```python
from build123d import *

# Parameters (mm, degrees)
CROQUIS1_W              = 167.894
CROQUIS1_H              = 52.07
SALIENTE_EXTRUIR1_DEPTH = 25.4
CROQUIS2_W              = 35
CROQUIS2_H              = 48.57
CORTAR_EXTRUIR1_DEPTH   = 25.4
CORTAR_EXTRUIR2_DEPTH   = 25.4
REDONDEO1_R             = 5
REDONDEO2_R             = 5
REDONDEO6_R             = 5
REDONDEO7_R             = 5
REDONDEO11_R            = 5
REDONDEO12_R            = 5
REDONDEO13_R            = 5
CROQUIS4_R              = 1.5
CORTAR_EXTRUIR3_DEPTH   = 76.2


with BuildPart() as part:
    # Croquis1 → Saliente-Extruir1 (new body)
    with BuildSketch(Plane.XY):
        with Locations((-83.947, 26.035)):
            Rectangle(CROQUIS1_W, CROQUIS1_H)
    extrude(amount=SALIENTE_EXTRUIR1_DEPTH)

    # Croquis2 → Cortar-Extruir1 (cut)
    with BuildSketch(Plane.XY.offset(25.4)):
        Polygon((-119.137953593, 52.07), (-132.894, 52.07), (-132.894, 3.5), (-120.129227268, 48.57), align=None)
        with Locations((-150.394, 27.785)):
            Rectangle(CROQUIS2_W, CROQUIS2_H)
        with Locations((-17.5, 27.785)):
            Rectangle(CROQUIS2_W, CROQUIS2_H)
        Polygon((-35, 52.07), (-48.756046407, 52.07), (-47.764772732, 48.57), (-35, 3.5), align=None)
    extrude(amount=-CORTAR_EXTRUIR1_DEPTH, mode=Mode.SUBTRACT)

    # Croquis3 → Cortar-Extruir2 (cut)
    with BuildSketch(Plane.XY.offset(25.4)):
        Polygon((-117.509109836, 48.57), (-50.384890164, 48.57), (-38.5, 3.5), (-38.5, 0), (-129.394, 0), (-129.394, 3.5), align=None)
    extrude(amount=-CORTAR_EXTRUIR2_DEPTH, mode=Mode.SUBTRACT)

    # Redondeo1
    redondeo1_edges = [part.edges().sort_by_distance(p)[0] for p in [
        (-48.756046407, 52.07, 12.7),
    ]]
    fillet(redondeo1_edges, radius=REDONDEO1_R)

    # Redondeo2
    redondeo2_edges = [part.edges().sort_by_distance(p)[0] for p in [
        (-119.137953593, 52.07, 12.7),
    ]]
    fillet(redondeo2_edges, radius=REDONDEO2_R)

    # Redondeo6
    redondeo6_edges = [part.edges().sort_by_distance(p)[0] for p in [
        (-38.5, 3.5, 12.7),
    ]]
    fillet(redondeo6_edges, radius=REDONDEO6_R)

    # Redondeo7
    redondeo7_edges = [part.edges().sort_by_distance(p)[0] for p in [
        (-129.394, 3.5, 12.7),
    ]]
    fillet(redondeo7_edges, radius=REDONDEO7_R)

    # Redondeo11
    redondeo11_edges = [part.edges().sort_by_distance(p)[0] for p in [
        (-129.394, 0, 12.7),
    ]]
    fillet(redondeo11_edges, radius=REDONDEO11_R)

    # Redondeo12
    redondeo12_edges = [part.edges().sort_by_distance(p)[0] for p in [
        (-38.5, 0, 12.7),
    ]]
    fillet(redondeo12_edges, radius=REDONDEO12_R)

    # Redondeo13
    redondeo13_edges = [part.edges().sort_by_distance(p)[0] for p in [
        (-132.894, 3.5, 12.7),
        (-35, 3.5, 12.7),
    ]]
    fillet(redondeo13_edges, radius=REDONDEO13_R)

    # Croquis4 → Cortar-Extruir3 (cut)
    with BuildSketch(Plane(origin=(0, 52.07, 0), x_dir=(1, 0, 0), z_dir=(0, 1, 0))):
        with Locations((-157.894, -5)):
            Circle(CROQUIS4_R)
        with Locations((-146.674562343, -20.4)):
            Circle(CROQUIS4_R)
        with Locations((-21.219437657, -20.4)):
            Circle(CROQUIS4_R)
        with Locations((-10, -5)):
            Circle(CROQUIS4_R)
    extrude(amount=-CORTAR_EXTRUIR3_DEPTH, mode=Mode.SUBTRACT)


solid = part.part
```
Geometry: final body of the model. Coordinates: model frame, mm. A direction names the side the tool comes from. Round coordinates to 2 decimals unless told otherwise and drop trailing zeros. Write each loop counter-clockwise with the first axis right and the second up, starting at its lowest first coordinate (ties: lowest second). Pieces come first, ordered by that corner, then holes. Notation, with made-up numbers: (49.25, 37.5) -> (90.25, 37.5) arc R17 ccw to (90.25, 63.5) -> close; hole circle Ø1 at (33, 25). An arc over 180 degrees is marked (long way). Return JSON: item names as keys, results as strings.
Q1. Section D-D on x = -63. Return the cut outline in (y, z), and give its area (3 significant figures).
From the geometry:
{"outline": "(48.57, 0) -> (52.07, 0) -> (52.07, 25.4) -> (48.57, 25.4) -> close", "area": "88.9 mm2"}
Q2. Section A-A on x = -10. Return the cut outline in (y, z).
From the geometry:
{"outline": "(0, 0) -> (3.5, 0) -> (3.5, 3.5) -> (0, 3.5) -> close; (0, 6.5) -> (3.5, 6.5) -> (3.5, 25.4) -> (0, 25.4) -> close"}
Q3. Section C-C on z = 20.4. Give the number of separate pieces and of enclosed holes in the cut face, and give its area (3 significant figures).
From the geometry:
{"separate pieces": "3", "enclosed holes": "0", "area": "765 mm2"}
Q4. First-contact query: pin 1 Ø5 at (x, z) = (-108.5, 17.5) entering from -Y; pin 2 Ø7.5 at (x, z) = (-158.5, 11.5) entering from +Y; pin 3 Ø3 at (x, y) = (-78, 46.5) entering from -Z. Flat tips, straight axial feed; report the tip coordinate or a pass-through.
From the geometry:
{"pin 1": "y = 48.57", "pin 2": "y = 3.5", "pin 3": "through"}
Q5. Set-up query: faces 5 (the flat face through (-153, 3.5, 13)), 6 (the flat face through (-123.45, 26.04, 12.88)), 7 (the flat face through (-16, 3.5, 13)). Return all of +Z, -Z, +X, -X, +Y, -Y with unobstructed straight access to the full face (end or side cutting, diameter ignored); none if empty.
From the geometry:
{"face 5": "+Z, -Z, -X, +Y", "face 6": "+Z, -Z, -Y", "face 7": "+Z, -Z, +X, +Y"}
Q6. Mould query, pull axis Z, two halves, no side actions, for faces 1 (the flat face through (-41.96, 28.07, 12.88)), 2 (the flat face through (-84, 49, 25.4)), 3 (the cylindrical face through (-148.173, 1.775, 20.334)), 4 (the cylindrical face through (-156.508, 1.775, 5.575)). Classes: +Z half, -Z half, draft (parallel to the pull), parting line (faces both ways), or undercut.
From the geometry:
{"face 1": "draft", "face 2": "+Z half", "face 3": "undercut", "face 4": "undercut"}
Q7. Ray query, line 1 (X direction, y = 1.15, z = 5); line 2 (X direction, y = 2.1, z = 20.4); line 3 (X direction, y = 13, z = 15.5). Return the intervals inside material, ascending.
From the geometry:
{"line 1": "-167.89 to -159.39, -156.39 to -130.97, -36.92 to -11.5, -8.5 to 0", "line 2": "-167.89 to -148.17, -145.17 to -130.09, -37.81 to -22.72, -19.72 to 0", "line 3": "-130.2 to -126.89, -41.01 to -37.69"}
Q8. Section B-B on y = 15.5. Return the cut outline in (x, z), and give its area (3 significant figures).
From the geometry:
{"outline": "(-129.5, 0) -> (-126.23, 0) -> (-126.23, 25.4) -> (-129.5, 25.4) -> close; (-41.66, 0) -> (-38.4, 0) -> (-38.4, 25.4) -> (-41.66, 25.4) -> close", "area": "166 mm2"}
